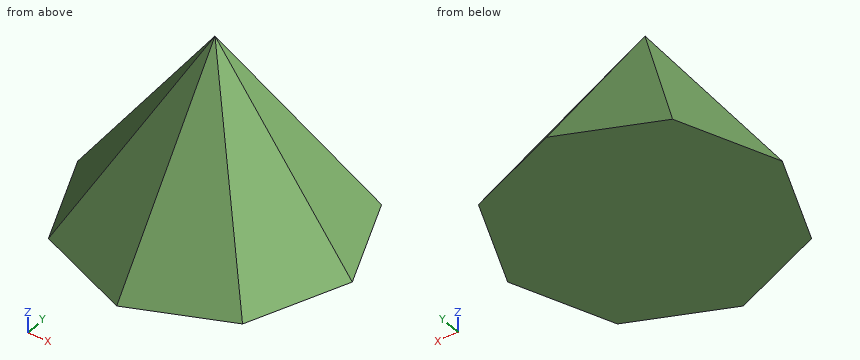
```python
from build123d import *


with BuildPart() as f3:
    # F0 (on Top) → F3 section 0
    with BuildSketch(Plane.XY, mode=Mode.PRIVATE) as f3_s0:
        Polygon((50.738705, 50.738705), (0, 71.755365), (-50.738705, 50.738705), (-71.755365, 0), (-50.738705, -50.738705), (0, -71.755365), (50.738705, -50.738705), (71.755365, 0), align=None)
    loft([Vertex(0, 0, 100), f3_s0.sketch])


solid = f3.part
```
Geometry: final body of the model. Coordinates: model frame, mm. Coordinates: 2 decimals unless noted, no trailing zeros. Write each loop counter-clockwise with the first axis right and the second up, starting at its lowest first coordinate (ties: lowest second). Pieces come first, ordered by that corner, then holes. Notation, with made-up numbers: M 29.25,71.25 L 69.25,71.25 A16 cw 69.25,98.25 Z; hole C 23.25,63.25 d11. An arc over 180 degrees is marked long. Answer as CSV lines item,"result". Start each with the question number.
Q1. Pin query (flat end, axial travel): P1, Ø2, axis at x = 3, z = 85.5, coming from the -Y side; P2, Ø6, axis at y = -34, z = 26.5, coming from the -X side; P3, Ø4, axis at x = -30.5, z = 10.5, coming from the -Y side. Return the tip coordinate at first contact, or that it passes through.
Q2. Cut plane A-A on z = 83. Return the cut outline in (x, y), then the cut area to 3 significant figures.
Q3. Cut plane D-D on z = 15.5. Return the cut outline in (x, y), then the cut area to 3 significant figures.
Q4. Line query: line 1 (Y direction, x = -2, z = 6); line 2 (Y direction, x = -29, z = 25.5); line 3 (Z direction, x = -27, y = -8). Output: solid intervals per line, ascending. Write a range as from..to.
Q5. Cut plane C-C on y = -19. Return the cut outline in (x, z), then the cut area to 3 significant figures.
Q6. Cut plane B-B on x = 12. Return the cut outline in (y, z).
Findings below:
1,P1,"stops at y = -9.99"
1,P2,"stops at x = -41.14"
1,P3,"stops at y = -53.24"
2,outline,"M -12.2,0 L -8.63,-8.63 L 0,-12.2 L 8.63,-8.63 L 12.2,0 L 8.63,8.63 L 0,12.2 L -8.63,8.63 Z"
2,area,"421 mm2"
3,outline,"M -60.63,0 L -42.87,-42.87 L 0,-60.63 L 42.87,-42.87 L 60.63,0 L 42.87,42.87 L 0,60.63 L -42.87,42.87 Z"
3,area,"10,400 mm2"
4,line 1,"y = -66.62..66.62"
4,line 2,"y = -41.45..41.45"
4,line 3,"z = 0..57.75"
5,outline,"M -63.89,0 L 63.89,0 L 19,62.55 L 0,73.52 L -19,62.55 Z"
5,area,"5,390 mm2"
6,outline,"M -66.78,0 L 66.78,0 L 12,76.35 L 0,83.28 L -12,76.35 Z"
